```python
from build123d import *

# Parameters (mm, degrees)
EXTRUDE_1_DEPTH          = 1.75
EXTRUDE_1_DEPTH_BACK     = 1.75
SKETCH_1_W               = 15
SKETCH_1_H               = 15
EXTRUDE_2_DEPTH          = 1
EXTRUDE_2_DEPTH_BACK     = 1
SKETCH_2_R               = 4.5
EXTRUDE_3_DEPTH          = 1.75
EXTRUDE_3_DEPTH_BACK     = 1.75
SKETCH_3_W               = 17.5
SKETCH_3_H               = 9.5
SKETCH_4_R               = 5
SKETCH_5_R               = 1
SKETCH_6_W               = 8
SKETCH_6_H               = 2
CUT_EXTRUDE_1_DEPTH      = 6
SKETCH_7_W               = 1
SKETCH_7_H               = 2.8
CUT_EXTRUDE_2_DEPTH      = 6
SKETCH_8_R               = 0.1
EXTRUDE_4_DEPTH          = 5
MIRROR_3_COPY_1_SKETCH_R = 0.1
MIRROR_3_COPY_1_DEPTH    = 5
FILLET_1_R               = 1.75
FILLET_2_R               = 0.2
FILLET_3_R               = 2


with BuildPart() as part:
    # 草图1 → 凸台-拉伸1 (new, two sides: drawn at the far end of the back side and taken through both)
    with BuildSketch(Plane(origin=(0, 0, 0), x_dir=(1, 0, 0), z_dir=(0, 1, 0)).offset(-EXTRUDE_1_DEPTH_BACK)):
        Rectangle(SKETCH_1_W, SKETCH_1_H)
    extrude(amount=EXTRUDE_1_DEPTH + EXTRUDE_1_DEPTH_BACK)

    # 草图2 → 凸台-拉伸2 (add, two sides: drawn at the far end of the back side and taken through both)
    with BuildSketch(Plane(origin=(0, 0, 0), x_dir=(1, 0, 0), z_dir=(0, 1, 0)).offset(-EXTRUDE_2_DEPTH_BACK)):
        with Locations((-7.5, 0)):
            Circle(SKETCH_2_R)
    extrude(amount=EXTRUDE_2_DEPTH + EXTRUDE_2_DEPTH_BACK)

    # 草图3 → 凸台-拉伸3 (add, two sides: drawn at the far end of the back side and taken through both)
    with BuildSketch(Plane(origin=(0, 0, 0), x_dir=(1, 0, 0), z_dir=(0, 1, 0)).offset(-EXTRUDE_3_DEPTH_BACK)):
        with Locations((16.25, 0)):
            Rectangle(SKETCH_3_W, SKETCH_3_H)
    extrude(amount=EXTRUDE_3_DEPTH + EXTRUDE_3_DEPTH_BACK)

    # 草图4 → 切除-放样1 section 0
    with BuildSketch(Plane(origin=(0, 1.75, 0), x_dir=(1, 0, 0), z_dir=(0, 1, 0))):
        Circle(SKETCH_4_R)
    # 草图5 → 切除-放样1 section 1
    with BuildSketch(Plane(origin=(0, 0.75, 0), x_dir=(1, 0, 0), z_dir=(0, 1, 0))):
        Circle(SKETCH_5_R)
    loft_1 = loft(mode=Mode.SUBTRACT)

    # 镜向1: 切除-放样1 across plane
    add(loft_1.mirror(Plane.ZX), mode=Mode.SUBTRACT)

    # 草图6 → 切除-拉伸1 (cut)
    with BuildSketch(Plane(origin=(25, 0, 0), x_dir=(0, 0, -1), z_dir=(1, 0, 0))):
        Rectangle(SKETCH_6_W, SKETCH_6_H)
    extrude(amount=-CUT_EXTRUDE_1_DEPTH, mode=Mode.SUBTRACT)

    # 草图7 → 切除-拉伸2 (cut)
    with BuildSketch(Plane(origin=(25, 0, 0), x_dir=(0, 0, -1), z_dir=(1, 0, 0))):
        Rectangle(SKETCH_7_W, SKETCH_7_H)
    extrude(amount=-CUT_EXTRUDE_2_DEPTH, mode=Mode.SUBTRACT)

    # 草图8 → 凸台-拉伸4 (add)
    with BuildSketch(Plane(origin=(19, 0, 0), x_dir=(0, 0, -1), z_dir=(1, 0, 0))):
        with Locations((-1.75, -1)):
            Circle(SKETCH_8_R)
    extrude_4 = extrude(amount=EXTRUDE_4_DEPTH)

    # 镜向2: 凸台-拉伸4 across plane
    add(extrude_4.mirror(Plane.XY))

    # 镜向3: 凸台-拉伸4 across plane
    add(extrude_4.mirror(Plane.ZX))

    # 镜向3 copy 1 sketch → 镜向3 copy 1 (add)
    with BuildSketch(Plane(origin=(19, 0, 0), x_dir=(0, 0, 1), z_dir=(1, 0, 0))):
        with Locations((-1.75, -1)):
            Circle(MIRROR_3_COPY_1_SKETCH_R)
    extrude(amount=MIRROR_3_COPY_1_DEPTH)

    # 圆角1
    fillet_1_edges = [part.edges().sort_by_distance(p)[0] for p in [
        (25, 1.2, 0.5),
        (25, 1.2, -0.5),
        (25, -1.2, -0.5),
        (25, -1.2, 0.5),
    ]]
    fillet(fillet_1_edges, radius=FILLET_1_R)

    # 圆角2
    fillet_2_edges = [part.edges().sort_by_distance(p)[0] for p in [
        (-7.5, -1.75, 0),
        (0, -1.75, 7.5),
        (0, -1.75, -7.5),
        (7.5, -1.75, -6.125),
        (7.5, -1.75, 6.125),
        (16.25, 1.75, 4.75),
        (16.25, -1.75, 4.75),
        (16.25, 1.75, -4.75),
        (16.25, -1.75, -4.75),
        (7.5, 1.75, 6.125),
        (7.5, 1.75, -6.125),
        (0, 1.75, -7.5),
        (0, 1.75, 7.5),
        (-7.5, 1.75, 0),
    ]]
    fillet(fillet_2_edges, radius=FILLET_2_R)

    # 圆角3
    # the kernel refuses this fillet: 2 mm, written as the material it takes off along each edge
    with BuildSketch(Plane(origin=(5.5, -1.75, -5.5), x_dir=(0, 0, -1), z_dir=(-1, 0, 0))) as fillet_3_piece_1:
        with BuildLine():
            CenterArc((1.8, -0.2), 0.2, 0, 90)
            Line((2, -0.2), (2, 0))
            Line((2, 0), (1.8, 0))
        make_face()
    revolve(axis=Axis((5.5, -1.75, -5.5), (0, -1, 0)), revolution_arc=90, mode=Mode.SUBTRACT)
    with BuildSketch(Plane(origin=(5.5, -1.75, 5.5), x_dir=(1, 0, 0), z_dir=(0, 0, -1))) as fillet_3_piece_2:
        with BuildLine():
            CenterArc((1.8, -0.2), 0.2, 0, 90)
            Line((2, -0.2), (2, 0))
            Line((2, 0), (1.8, 0))
        make_face()
    revolve(axis=Axis((5.5, -1.75, 5.5), (0, -1, 0)), revolution_arc=90, mode=Mode.SUBTRACT)
    with BuildSketch(Plane(origin=(-5.5, -1.75, -5.5), x_dir=(-1, 0, 0), z_dir=(0, 0, 1))) as fillet_3_piece_3:
        with BuildLine():
            CenterArc((1.8, -0.2), 0.2, 0, 90)
            Line((2, -0.2), (2, 0))
            Line((2, 0), (1.8, 0))
        make_face()
    revolve(axis=Axis((-5.5, -1.75, -5.5), (0, -1, 0)), revolution_arc=90, mode=Mode.SUBTRACT)
    with BuildSketch(Plane(origin=(-5.5, -1.75, 5.5), x_dir=(0, 0, 1), z_dir=(1, 0, 0))) as fillet_3_piece_4:
        with BuildLine():
            CenterArc((1.8, -0.2), 0.2, 0, 90)
            Line((2, -0.2), (2, 0))
            Line((2, 0), (1.8, 0))
        make_face()
    revolve(axis=Axis((-5.5, -1.75, 5.5), (0, -1, 0)), revolution_arc=90, mode=Mode.SUBTRACT)
    with BuildSketch(Plane(origin=(5.5, 1.75, -5.5), x_dir=(1, 0, 0), z_dir=(0, 0, 1))) as fillet_3_piece_5:
        with BuildLine():
            CenterArc((1.8, -0.2), 0.2, 0, 90)
            Line((2, -0.2), (2, 0))
            Line((2, 0), (1.8, 0))
        make_face()
    revolve(axis=Axis((5.5, 1.75, -5.5), (0, 1, 0)), revolution_arc=90, mode=Mode.SUBTRACT)
    with BuildSketch(Plane(origin=(-5.5, 1.75, -5.5), x_dir=(0, 0, -1), z_dir=(1, 0, 0))) as fillet_3_piece_6:
        with BuildLine():
            CenterArc((1.8, -0.2), 0.2, 0, 90)
            Line((2, -0.2), (2, 0))
            Line((2, 0), (1.8, 0))
        make_face()
    revolve(axis=Axis((-5.5, 1.75, -5.5), (0, 1, 0)), revolution_arc=90, mode=Mode.SUBTRACT)
    with BuildSketch(Plane(origin=(-5.5, 1.75, 5.5), x_dir=(-1, 0, 0), z_dir=(0, 0, -1))) as fillet_3_piece_7:
        with BuildLine():
            CenterArc((1.8, -0.2), 0.2, 0, 90)
            Line((2, -0.2), (2, 0))
            Line((2, 0), (1.8, 0))
        make_face()
    revolve(axis=Axis((-5.5, 1.75, 5.5), (0, 1, 0)), revolution_arc=90, mode=Mode.SUBTRACT)
    with BuildSketch(Plane(origin=(5.5, 1.75, 5.5), x_dir=(0, 0, 1), z_dir=(-1, 0, 0))) as fillet_3_piece_8:
        with BuildLine():
            CenterArc((1.8, -0.2), 0.2, 0, 90)
            Line((2, -0.2), (2, 0))
            Line((2, 0), (1.8, 0))
        make_face()
    revolve(axis=Axis((5.5, 1.75, 5.5), (0, 1, 0)), revolution_arc=90, mode=Mode.SUBTRACT)
    with BuildSketch(Plane(origin=(-7.5, 1.75, 7.5), x_dir=(1, 0, 0), z_dir=(0, -1, 0)), Plane(origin=(-7.5, -1.75, -7.5), x_dir=(1, 0, 0), z_dir=(0, 1, 0)), Plane(origin=(7.5, 1.75, 7.5), x_dir=(0, 0, -1), z_dir=(0, -1, 0)), Plane(origin=(7.5, -1.75, -7.5), x_dir=(0, 0, 1), z_dir=(0, 1, 0))) as fillet_3_piece_9:
        with BuildLine():
            CenterArc((FILLET_3_R, -FILLET_3_R), FILLET_3_R, 90, 90)
            Line((0, -FILLET_3_R), (0, 0))
            Line((0, 0), (FILLET_3_R, 0))
        make_face()
    extrude(amount=3.5, mode=Mode.SUBTRACT)


solid = part.part
```
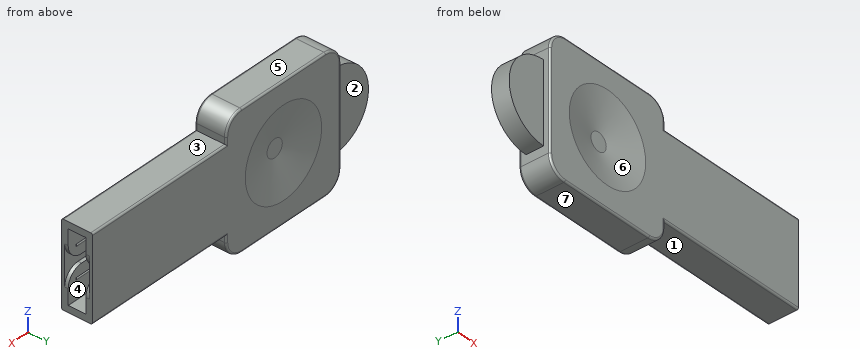
Design review of the part built by this model. Coordinates are the model's own, in mm. Face numbers are marked on the shaded views. A direction names the side the tool comes from. Give positions to 0.01 mm unless a question says otherwise; leave off trailing zeros. Loops run counter-clockwise (first coordinate to the right, second up) from the corner with the lowest first, then second, coordinate; pieces in that order, holes last. Notation, with made-up numbers: M 32.25,4 L 49.25,4 A21 ccw 49.25,24 Z; hole C 75.5,59.5 d7. An arc over 180 degrees is marked long. Return JSON: item names as keys, results as strings. Group by question number.
Item 1: Tool access review of the marked faces 1, 2, 3 and 4: name each direction out of +Z, -Z, +X, -X, +Y, -Y from which nothing blocks a thin tool from reaching the whole face with its end or side.
Item 2: For probe 1 along Z at (x, y) = (11.5, 0.7); probe 2 along X at (y, z) = (-1.25, 5.5); probe 3 along X at (y, z) = (-1.4, 4.5), list the stretches that pass through material, from the lowest coordinate up.
Item 3: We need section D-D (x = 0). Give the boundary of the cut face in (y, z), and give its area (3 significant figures).
Item 4: Insertion check: pin 1 Ø2 at (x, z) = (-9.5, -2) entering from +Y; pin 2 Ø2 at (x, y) = (22.5, 0) entering from +Z; pin 3 Ø1.6 at (x, z) = (0.5, 0) entering from +Y (3 decimals). Each pin has a flat end and moves straight along its axis. Give the tip position at first contact, or say it passes through.
Item 5: We need section C-C (x = 21). Give the boundary of the cut face in (y, z).
Item 6: We need section B-B (y = 0.35). Give the boundary of the cut face in (x, z), and give its area (3 significant figures).
Item 7: We need section A-A (x = 14). Give the boundary of the cut face in (y, z), and give its area (3 significant figures).
Item 8: Mouldability with a two-part tool opening along Z and no side actions: class the marked faces 5, 6 and 7 as released by +Z, released by -Z, zero draft, split by the parting line, or undercut.
Output:
{
 "1": {"face 1": "-Z, +X, +Y, -Y", "face 2": "+Z, -Z, -X, +Y", "face 3": "+Z, +X, +Y, -Y", "face 4": "+X"},
 "2": {"probe 1": "z = -4.75 to 4.75", "probe 2": "x = -7.5 to 7.5", "probe 3": "x = -7.5 to 25"},
 "3": {"outline": "M -1.75,-7.3 A0.2 ccw -1.55,-7.5 L 1.55,-7.5 A0.2 ccw 1.75,-7.3 L 1.75,-5 L 0.75,-1 L 0.75,1 L 1.75,5 L 1.75,7.3 A0.2 ccw 1.55,7.5 L -1.55,7.5 A0.2 ccw -1.75,7.3 L -1.75,5 L -0.75,1 L -0.75,-1 L -1.75,-5 Z", "area": "40.5 mm^2"},
 "4": {"pin 1": "stops at y = 1", "pin 2": "stops at z = 4.75", "pin 3": "stops at y = 0.825"},
 "5": {"outline": "M -1.75,-4.55 A0.2 ccw -1.55,-4.75 L 1.55,-4.75 A0.2 ccw 1.75,-4.55 L 1.75,4.55 A0.2 ccw 1.55,4.75 L -1.55,4.75 A0.2 ccw -1.75,4.55 Z; hole M -1.4,-0.5 L -1,-0.5 L -1,-1.65 A0.1 cw -1,-1.85 L -1,-4 L 1,-4 L 1,-1.85 A0.1 cw 1,-1.65 L 1,-0.5 L 1.4,-0.5 L 1.4,0.5 L 1,0.5 L 1,1.65 A0.1 cw 1,1.85 L 1,4 L -1,4 L -1,1.85 A0.1 cw -1,1.65 L -1,0.5 L -1.4,0.5 Z"},
 "6": {"outline": "M -7.5,-5.5 A2 ccw -5.5,-7.5 L 5.5,-7.5 A2 ccw 7.5,-5.5 L 7.5,-4.75 L 25,-4.75 L 25,-4 L 19,-4 L 19,4 L 25,4 L 25,4.75 L 7.5,4.75 L 7.5,5.5 A2 ccw 5.5,7.5 L -5.5,7.5 A2 ccw -7.5,5.5 L -7.5,4.5 A4.5 ccw -7.5,-4.5 Z", "area": "372 mm^2"},
 "7": {"outline": "M -1.75,-4.55 A0.2 ccw -1.55,-4.75 L 1.55,-4.75 A0.2 ccw 1.75,-4.55 L 1.75,4.55 A0.2 ccw 1.55,4.75 L -1.55,4.75 A0.2 ccw -1.75,4.55 Z", "area": "33.2 mm^2"},
 "8": {"face 5": "released by +Z", "face 6": "undercut", "face 7": "released by -Z"}
}
